```python
from build123d import *

# Parameters (mm, degrees)
F0_W     = 50.8
F0_H     = 1.668666
F0_H_2   = 99.931334
F1_DEPTH = 1.524
F2_DEPTH = 33.274
F3_W     = 42.008801
F3_H     = 2.4892
F4_DEPTH = 33.274
F5_R     = 12.446
F6_DEPTH = 25.4
F7_R     = 3.656717
F8_DEPTH = 25.4


with BuildPart() as f1:
    # F0 (on Top) → F1 (new body)
    with BuildSketch(Plane.XY):
        with Locations((-13.704186, 132.995608)):
            Rectangle(F0_W, F0_H)
        with Locations((-13.704186, 82.195608)):
            Rectangle(F0_W, F0_H_2)
    extrude(amount=F1_DEPTH)

    # F0 (on Top) → F2 (join)
    with BuildSketch(Plane.XY):
        with Locations((-13.704186, 132.995608)):
            Rectangle(F0_W, F0_H)
    extrude(amount=F2_DEPTH)

    # F3 (on face) → F4 (join)
    with BuildSketch(Plane(origin=(0, 133.829941, 0), x_dir=(-1, 0, 0), z_dir=(0, 1, 0))):
        with Locations((14.214616, 32.0294)):
            Rectangle(F3_W, F3_H)
    extrude(amount=F4_DEPTH)

    # F5 (on face) → F6 (cut)
    with BuildSketch(Plane.XY.offset(33.274)):
        with Locations((-17.118977, 146.331966)):
            Circle(F5_R)
    extrude(amount=-F6_DEPTH, mode=Mode.SUBTRACT)

    # F7 (on face) → F8 (join)
    with BuildSketch(Plane(origin=(0, 0, 30.7848), x_dir=(1, 0, 0), z_dir=(0, 0, -1))):
        with Locations((-15.556242, -163.017869)):
            Circle(F7_R)
    extrude(amount=F8_DEPTH)


solid = f1.part
```
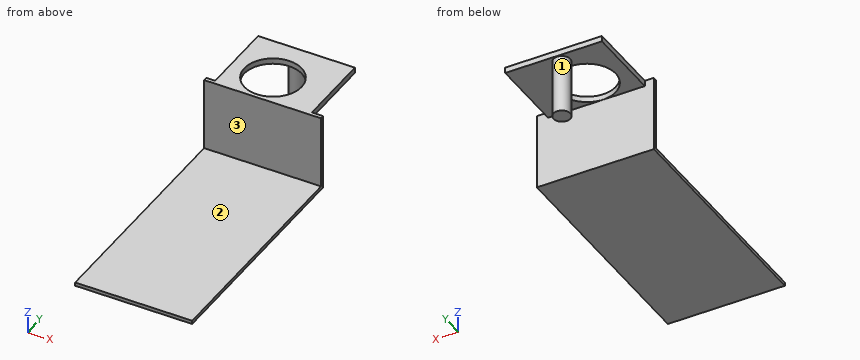
Design review of the part built by this model. Coordinates are the model's own, in mm. Face numbers are marked on the shaded views. Coordinates: 2 decimals unless noted, no trailing zeros. Order: outer loops, then holes, each group sorted by start corner. A loop starts at its lowest first (then second) coordinate and runs counter-clockwise, first axis right, second up. Notation, with made-up numbers: M 47,81 L 87,81 A22 cw 87,113 Z; hole C 13.5,14.5 d9. An arc over 180 degrees is marked long. Answer as a JSON object with one key per item and string values. Group by question number.
1) Mouldability with a two-part tool opening along Y and no side actions: class the marked faces 1, 2 and 3 as pulls with the +Y half, pulls with the -Y half, needs draft (parallel to the pull), parting line crosses it, or undercut.
2) For pin 1 (2.5 mm diameter, centred on y = 151.5, z = 32.5, fed in from +X); pin 2 (0.7 mm diameter, centred on y = 145, z = 32, fed in from -X); pin 3 (2 mm diameter, centred on x = -26.5, y = 102, fed in from +Z); pin 4 (6 mm diameter, centred on x = 1, z = 28.5, fed in from +Y), all flat-tipped, find the tip position at first contact; note any pin that passes through.
3) Wall thickness on L1, parallel to Y at x = -7, z = 25; L2, parallel to Z at x = -21.5, y = 89; L3, parallel to Z at x = -8, y = 160.5: over which ranges is each line inside the solid? List them lowest first.
4) Add section B-B, the plane x = 3. Write out the cut boundary in (y, z).
5) Add section D-D, the plane z = 20. Write out the cut boundary in (x, y).
6) Add section C-C, the plane y = 149.5. Write out the cut boundary in (x, z).
7) Add section A-A, the plane x = -21. Write out the cut boundary in (y, z), then the cut area to 3 significant figures.
Computed values:
{
 "1": {"face 1": "undercut", "face 2": "needs draft", "face 3": "pulls with the -Y half"},
 "2": {"pin 1": "stops at x = 6.79", "pin 2": "stops at x = -35.22", "pin 3": "stops at z = 1.52", "pin 4": "stops at y = 167.1"},
 "3": {"L1": "y = 132.16 to 133.83", "L2": "z = 0 to 1.52", "L3": "z = 30.78 to 33.27"},
 "4": {"outline": "M 32.23,0 L 133.83,0 L 133.83,30.78 L 167.1,30.78 L 167.1,33.27 L 132.16,33.27 L 132.16,1.52 L 32.23,1.52 Z"},
 "5": {"outline": "M -39.1,132.16 L 11.7,132.16 L 11.7,133.83 L -39.1,133.83 Z; C -15.56,163.02 d7.31"},
 "6": {"outline": "M -35.22,30.78 L -29.16,30.78 L -29.16,33.27 L -35.22,33.27 Z; M -5.08,30.78 L 6.79,30.78 L 6.79,33.27 L -5.08,33.27 Z"},
 "7": {"outline": "M 32.23,0 L 133.83,0 L 133.83,30.78 L 134.51,30.78 L 134.51,33.27 L 132.16,33.27 L 132.16,1.52 L 32.23,1.52 Z; M 158.16,30.78 L 167.1,30.78 L 167.1,33.27 L 158.16,33.27 Z", "area": "232 mm^2"}
}
